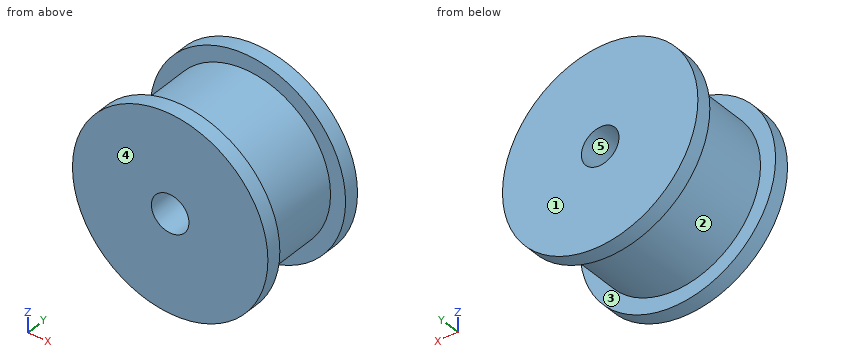
from build123d import *

# Parameters (mm, degrees)
SKETCH_1_R      = 13
EXTRUDE_1_DEPTH = 2
SKETCH_2_R      = 11
EXTRUDE_2_DEPTH = 11
SKETCH_3_R      = 13
EXTRUDE_3_DEPTH = 2
HOLE_WIZARD_1_D = 5


with BuildPart() as part:
    # 草图1 → 凸台-拉伸1 (new body)
    with BuildSketch(Plane(origin=(0, 0, 0), x_dir=(1, 0, 0), z_dir=(0, 1, 0))):
        with Locations(Location((0, 0, 0), (0, 0, 270))):
            Circle(SKETCH_1_R)
    extrude(amount=EXTRUDE_1_DEPTH)

    # 草图2 → 凸台-拉伸2 (add)
    with BuildSketch(Plane(origin=(0, 2, 0), x_dir=(1, 0, 0), z_dir=(0, 1, 0))):
        with Locations(Location((0, 0, 0), (0, 0, 270))):
            Circle(SKETCH_2_R)
    extrude(amount=EXTRUDE_2_DEPTH)

    # 草图3 → 凸台-拉伸3 (add)
    with BuildSketch(Plane(origin=(0, 13, 0), x_dir=(1, 0, 0), z_dir=(0, 1, 0))):
        with Locations(Location((0, 0, 0), (0, 0, 270))):
            Circle(SKETCH_3_R)
    extrude(amount=EXTRUDE_3_DEPTH)

    # 孔1 (through all)
    with Locations(Plane(origin=(0, 15, 0), x_dir=(1, 0, 0), z_dir=(0, 1, 0))):
        with Locations((0, 0)):
            Hole(HOLE_WIZARD_1_D / 2)


solid = part.part
Build history of the part. All positions in model axes, mm. Face numbers are marked on the shaded views. A direction names the side the tool comes from. Give positions to 0.01 mm unless a question says otherwise; leave off trailing zeros. Loops run counter-clockwise (first coordinate to the right, second up) from the corner with the lowest first, then second, coordinate; pieces in that order, holes last. Notation, with made-up numbers: (89.5, 2.5) - (145.5, 2.5) arc R23 ccw to (145.5, 33.5) - close; hole circle Ø10 at (44.25, 70). An arc over 180 degrees is marked (long way). Write item = value, one per line. Start each with the question number.
1) Band-saw the part on C-C on y = 11. Give the cut face in (x, z), plus the area to 3 significant figures.
2) Band-saw the part on D-D on x = -10.5. Give the cut face in (y, z).
3) Tool access for the marked faces 1 and 2: list every direction of +Z, -Z, +X, -X, +Y, -Y with a clear straight run to the whole face (end or side of a thin tool).
4) Band-saw the part on B-B on z = 0. Give the cut face in (x, y).
5) Pull direction Y, two halves, no side cores. Call the marked faces 3, 4 and 5: +Y half, -Y half, draft (parallel to the pull), parting line (faces both ways), or undercut.
6) Drop flat-ended pins along their axis: pin 1 Ø5 at (y, z) = (3, 3.5) entering from -X; pin 2 Ø4 at (y, z) = (7, 4.5) entering from -X; pin 3 Ø1 at (y, z) = (4, 8) entering from +X. Give the stop position or say it passes through.
7) Probe probe 1 along Y at (x, z) = (10, -8); probe 2 along Z at (x, y) = (-1.25, 4.5); probe 3 along Z at (x, y) = (1.5, 12.5). List the from-to ranges inside material, lowest first. Write a range as from..to.
8) Band-saw the part on A-A on x = 0. Give the cut face in (y, z), plus the area to 3 significant figures.
Final values:
q1.outline = circle Ø22 at (0, 0); hole circle Ø5 at (0, 0)
q1.area = 360 mm²
q2.outline = (0, -7.66) - (2, -7.66) - (2, -3.28) - (13, -3.28) - (13, -7.66) - (15, -7.66) - (15, 7.66) - (13, 7.66) - (13, 3.28) - (2, 3.28) - (2, 7.66) - (0, 7.66) - close
q3.face_1 = +Z, -Z, +X, -X, +Y
q3.face_2 = none
q4.outline = (-13, 0) - (-2.5, 0) - (-2.5, 15) - (-13, 15) - (-13, 13) - (-11, 13) - (-11, 2) - (-13, 2) - close; (2.5, 0) - (13, 0) - (13, 2) - (11, 2) - (11, 13) - (13, 13) - (13, 15) - (2.5, 15) - close
q5.face_3 = undercut
q5.face_4 = -Y half
q5.face_5 = draft
q6.pin_1 = -12.94
q6.pin_2 = -10.71
q6.pin_3 = 8.05
q7.probe_1 = 0..2, 13..15
q7.probe_2 = -10.93..-2.17, 2.17..10.93
q7.probe_3 = -10.9..-2, 2..10.9
q8.outline = (0, -13) - (2, -13) - (2, -11) - (13, -11) - (13, -13) - (15, -13) - (15, -2.5) - (0, -2.5) - close; (0, 2.5) - (15, 2.5) - (15, 13) - (13, 13) - (13, 11) - (2, 11) - (2, 13) - (0, 13) - close
q8.area = 271 mm²
